For this review, take the finished solid that the model builds, in its own axes (mm). Face numbers are marked on the shaded views. A direction names the side the tool comes from. Coordinates: 2 decimals unless noted, no trailing zeros. Loops run counter-clockwise (first coordinate to the right, second up) from the corner with the lowest first, then second, coordinate; pieces in that order, holes last.
1. Machinability: for the marked faces 5 and 6, which of the approach directions +Z, -Z, +X, -X, +Y, -Y give a long, thin tool a straight path to every point of the face, cutting with its end or side? Answer none if there is none.
2. To check wall thickness, follow probe 1 along Z at (x, y) = (19, -29); probe 2 along X at (y, z) = (-30, -11); probe 3 along Z at (x, y) = (-30.5, -5.5). State the ranges of each line that lie inside material, in increasing order.
3. Clearance check with flat-ended pins moving along their axes: P1, Ø10, axis at x = -7, y = -14, coming from the -Z side; P2, Ø5, axis at x = -10.5, z = 15.5, coming from the -Y side; P3, Ø12, axis at x = -18, z = -14.5, coming from the +Y side. State where each tip first meets the part, or that it passes through.
4. Take a section at B-B, the plane z = -1.5. State the section outline as (x, y) points, then the cut area to 3 significant figures.
5. Take a section at C-C, the plane y = -28. Count the separate pieces of the cut face and the enclosed holes in it, then the cut area to 3 significant figures.
6. Mouldability with a two-part tool opening along X and no side actions: class the marked faces 1, 2, 3 and 4 as pulls with the +X half, pulls with the -X half, needs draft (parallel to the pull), parting line crosses it, or undercut.
7. Take a section at A-A, the plane x = -20. State the section outline as (y, z) points, then the cut area to 3 significant figures.
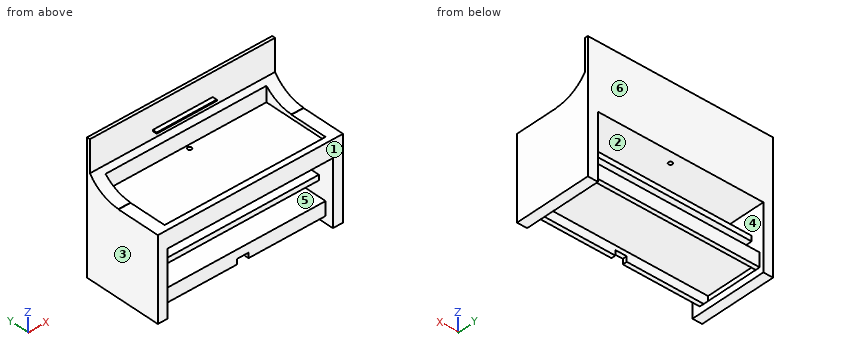
```python
from build123d import *

# Parameters (mm, degrees)
F0_W          = 109.3183457851
F0_H          = 33.4434658289
F1_DEPTH      = 45.72
F2_W          = 95.0407683849
F2_H          = 38.138333708
F3_DEPTH      = 25.4
F4_W          = 109.3183457851
F4_H          = 23.2531316578
F5_DEPTH      = 25.4
F7_DEPTH      = 254
F9_W          = 5.9644132853
F9_H          = 45.72
F9_W_2        = 5.7119317353
F10_DEPTH     = 38.1
F11_W         = 29.130092822
F11_H         = 3.0559636652
F12_DEPTH     = 101.6
F14_DEPTH     = 127
F15_DEPTH     = 18.5456499457
F16_W         = 35.4631710798
F16_H         = 0.6852131337
F17_DEPTH     = 2.54
F18_W         = 38.6509299278
F18_H         = 8.1171598285
F19_DEPTH     = 99.9768525362
F20_T         = 2.54
F20_T3_DEPTH  = 114.3983457851
F20_T5_DEPTH  = 40.5431710798
F20_T7_DEPTH  = 5.7652131337
F20_T9_DEPTH  = 12.2003224361
F20_T11_DEPTH = 12.2372549641
F20_T13_DEPTH = 50.8
F20_T15_DEPTH = 13.1971598285
F20_T17_DEPTH = 43.7309299278
F20_T19_DEPTH = 34.210092822
F20_T21_DEPTH = 8.1359636652
F20_T23_DEPTH = 7.2268683422
F20_T25_DEPTH = 43.218333708
F20_T27_DEPTH = 14.0249238314
F20_T29_DEPTH = 100.1207683849
F21_W         = 6.7161731422
F21_H         = 3.0271708965
F22_DEPTH     = 25.4
F8_R          = 1.1732121366
F23_DEPTH     = 69.3976804614


# Not quite as in the source:
# - a shell that OpenCascade refuses in one call is made with other operations: the cavity is built on its own and cut out


with BuildPart() as f1:
    # F0 (on Front) → F1 (new body)
    with BuildSketch(Plane.XZ):
        with Locations((-0.1045018435, 16.7217329144)):
            Rectangle(F0_W, F0_H)
    extrude(amount=F1_DEPTH)

    # F2 (on face) → F3 (cut)
    with BuildSketch(Plane.XY.offset(33.4434658289)):
        with Locations((-0.1229681075, -23.2116412371)):
            Rectangle(F2_W, F2_H)
    extrude(amount=-F3_DEPTH, mode=Mode.SUBTRACT)

    # F4 (on face) → F5 (cut)
    with BuildSketch(Plane.XZ.offset(45.72)):
        with Locations((-0.1045018435, 21.8169)):
            Rectangle(F4_W, F4_H)
    extrude(amount=-F5_DEPTH, mode=Mode.SUBTRACT)

    # F6 (on face) → F7 (cut)
    with BuildSketch(Plane.YZ.offset(54.5546710491)):
        with BuildLine():
            Line((-20.32, 33.4434658289), (-20.32, 10.3678972162))
            ThreePointArc((-20.32, 10.3678972162), (-8.4847772871, 13.6341404962), (0, 22.5082261516))
            Line((0, 22.5082261516), (0, 33.4434658289))
            Line((0, 33.4434658289), (-20.32, 33.4434658289))
        make_face()
        with BuildLine():
            ThreePointArc((0, 22.5082261516), (2.0560745106, 27.8049237926), (2.7555686127, 33.4434658289))
            ThreePointArc((2.7555686127, 33.4434658289), (-36.6368910458, 49.7603568747), (-20.32, 10.3678972162))
            Line((-20.32, 10.3678972162), (-20.32, 33.4434658289))
            Line((-20.32, 33.4434658289), (0, 33.4434658289))
            Line((0, 33.4434658289), (0, 22.5082261516))
        make_face()
    extrude(amount=-F7_DEPTH, mode=Mode.SUBTRACT)

    # F9 (on face) → F10 (join)
    with BuildSketch(Plane(origin=(0, 0, 0), x_dir=(1, 0, 0), z_dir=(0, 0, -1))):
        with Locations((51.5724644065, 22.86)):
            Rectangle(F9_W, F9_H)
        with Locations((-51.9077088684, 22.86)):
            Rectangle(F9_W_2, F9_H)
    extrude(amount=F10_DEPTH)

    # F11 (on face) → F12 (join)
    with BuildSketch(Plane.YZ.offset(-49.0517430007)):
        with Locations((-22.1103844233, -15.5687723309)):
            Rectangle(F11_W, F11_H)
    extrude(amount=F12_DEPTH)

    # F13 (on face) → F14 (cut)
    with BuildSketch(Plane.YZ.offset(54.5546710491)):
        with BuildLine():
            ThreePointArc((0, 22.5082261516), (-0.8668457158, 21.0315096899), (-1.8408102843, 19.6231397021))
            Line((-1.8408102843, 19.6231397021), (0, 19.6231397021))
            Line((0, 19.6231397021), (0, 22.5082261516))
        make_face()
    extrude(amount=-F14_DEPTH, mode=Mode.SUBTRACT)

    # F15 (add): a face of the model
    f15_faces = [f1.faces().sort_by_distance(p)[0] for p in [
        (-0.1045018435, -0.9204051421, 19.6231397021),
    ]]
    extrude(f15_faces, amount=F15_DEPTH)

    # F16 (on face) → F17 (join)
    with BuildSketch(Plane.XZ.offset(1.8408102843)):
        with Locations((0.1093326136, 24.1770995781)):
            Rectangle(F16_W, F16_H)
    extrude(amount=F17_DEPTH)

    # F18 (on face) → F19 (join)
    with BuildSketch(Plane(origin=(48.5902577639, 0, 0), x_dir=(0, -1, 0), z_dir=(-1, 0, 0))):
        with Locations((21.6686017811, -30.0215007737)):
            Rectangle(F18_W, F18_H)
    extrude(amount=F19_DEPTH)

    # F20: shell of thickness 2.54, made by hand


with BuildPart() as f20_core1:
    # F20_t2: copy of F1
    add(f1.part)

    # the walls: a layer under each face that stays
    f20_faces = [f20_core1.faces().sort_by_distance(p)[0] for p in [
        (-54.763674736, -22.86, 0.0343948239),
        (-0.1045018435, 0, 0.0343948239),
        (-0.1045018435, -0.9204051421, 38.1687896479),
        (-0.1045018435, -1.8408102843, 28.895964675),
        (-46.9552214657, -2.7975084588, 18.4286678952),
        (-51.203513518, -20.32, 10.2791156936),
        (-46.9552214657, -43.9057142857, 10.1903341711),
        (-36.5439504385, -45.72, 2.1419451425),
        (-51.9077088684, -22.86, -38.1),
        (54.5546710491, -22.86, 0.0343948239),
        (-49.0517430007, -22.86, -19.05),
        (-0.2307426184, -22.86, 0),
        (48.5902577639, -22.86, -19.05),
        (51.5724644065, -22.86, -38.1),
        (0.1093326136, -3.1108102843, 24.5197061449),
        (-17.6222529262, -3.1108102843, 24.1770995781),
        (0.1093326136, -3.1108102843, 23.8344930112),
        (17.8409181535, -3.1108102843, 24.1770995781),
        (-47.6433522999, -10.4988633345, 9.5342864675),
        (-0.1229681075, -4.1424743831, 12.5159277446),
        (47.397416085, -35.9244191398, 9.5342864675),
        (50.9760435671, -20.32, 10.2791156936),
        (-0.1229681075, -42.2808080912, 9.1169),
        (-0.2307426184, -40.994066745, -30.0215007737),
        (-0.2307426184, -21.6686017811, -25.9629208595),
        (-0.2307426184, -2.3431368172, -30.0215007737),
        (-0.2307426184, -22.1103844233, -14.0407904983),
        (-0.2307426184, -7.5453380123, -15.5687723309),
        (-0.2307426184, -36.6754308343, -15.5687723309),
        (-0.2307426184, -22.1103844233, -17.0967541635),
        (0.1093326136, -4.3808102843, 24.1770995781),
        (-0.1229681075, -23.2116412371, 8.0434658289),
    ]]
    thicken(f20_faces, amount=-F20_T, mode=Mode.SUBTRACT)

    # F20_s4 → F20_t3 (cut)
    with BuildSketch(Plane.YZ.offset(-57.303674736)):
        Polygon((-1.8865509063, 19.6383521673), (0.6991897157, 19.6231397021), (0.6991897157, 18.7783837759), (0.1932519166, 18.1018931859), align=None)
    extrude(amount=F20_T3_DEPTH, mode=Mode.SUBTRACT)

    # F20_s6 → F20_t5 (cut)
    with BuildSketch(Plane.YZ.offset(-20.1622529262)):
        Polygon((-1.8662102843, 24.5451061449), (0.6991897157, 24.5197061449), (0.6991897157, 21.9797061449), (-1.8408102843, 21.9797061449), align=None)
        Polygon((-1.8662102843, 23.8090930112), (0.6991897157, 23.8344930112), (0.6991897157, 26.3744930112), (-1.8408102843, 26.3744930112), align=None)
    extrude(amount=F20_T5_DEPTH, mode=Mode.SUBTRACT)

    # F20_s8 → F20_t7 (cut)
    with BuildSketch(Plane.XY.offset(21.2944930112)):
        Polygon((-17.6476529262, -1.8662102843), (-17.6222529262, 0.6991897157), (-15.0822529262, 0.6991897157), (-15.0822529262, -1.8408102843), align=None)
        Polygon((17.8663181535, -1.8662102843), (17.8409181535, 0.6991897157), (15.3009181535, 0.6991897157), (15.3009181535, -1.8408102843), align=None)
    extrude(amount=F20_T7_DEPTH, mode=Mode.SUBTRACT)

    # F20_s10 → F20_t9 (cut)
    with BuildSketch(Plane.YZ.offset(-57.303674736)):
        Polygon((-20.3454, 10.2157341711), (-17.78, 10.1903341711), (-17.78, 7.6503341711), (-20.32, 7.6503341711), align=None)
    extrude(amount=F20_T9_DEPTH, mode=Mode.SUBTRACT)

    # F20_s12 → F20_t11 (cut)
    with BuildSketch(Plane.YZ.offset(44.857416085)):
        Polygon((-20.3454, 10.2157341711), (-20.32, 7.6503341711), (-17.78, 7.6503341711), (-17.78, 10.1903341711), align=None)
    extrude(amount=F20_T11_DEPTH, mode=Mode.SUBTRACT)

    # F20_s14 → F20_t13 (cut)
    with BuildSketch(Plane.XZ.offset(-2.54)):
        Polygon((-49.0263430007, -0.0254), (-51.5917430007, 0), (-51.5917430007, 2.54), (-49.0517430007, 2.54), align=None)
        Polygon((48.5648577639, -0.0254), (48.5902577639, 2.54), (51.1302577639, 2.54), (51.1302577639, 0), align=None)
    extrude(amount=F20_T13_DEPTH, mode=Mode.SUBTRACT)

    # F20_s16 → F20_t15 (cut)
    with BuildSketch(Plane.XY.offset(-36.620080688)):
        Polygon((-49.0263430007, -41.019466745), (-51.5917430007, -40.994066745), (-51.5917430007, -38.454066745), (-49.0517430007, -38.454066745), align=None)
        Polygon((-49.0263430007, -2.3177368172), (-51.5917430007, -2.3431368172), (-51.5917430007, -4.8831368172), (-49.0517430007, -4.8831368172), align=None)
        Polygon((48.5648577639, -2.3177368172), (51.1302577639, -2.3431368172), (51.1302577639, -4.8831368172), (48.5902577639, -4.8831368172), align=None)
        Polygon((48.5648577639, -41.019466745), (51.1302577639, -40.994066745), (51.1302577639, -38.454066745), (48.5902577639, -38.454066745), align=None)
    extrude(amount=F20_T15_DEPTH, mode=Mode.SUBTRACT)

    # F20_s18 → F20_t17 (cut)
    with BuildSketch(Plane.XZ.offset(-0.1968631828)):
        Polygon((-49.0263430007, -25.9375208595), (-51.5917430007, -25.9629208595), (-51.5917430007, -28.5029208595), (-49.0517430007, -28.5029208595), align=None)
        Polygon((48.5648577639, -25.9375208595), (51.1302577639, -25.9629208595), (51.1302577639, -28.5029208595), (48.5902577639, -28.5029208595), align=None)
    extrude(amount=F20_T17_DEPTH, mode=Mode.SUBTRACT)

    # F20_s20 → F20_t19 (cut)
    with BuildSketch(Plane.XZ.offset(5.0053380123)):
        Polygon((-49.0263430007, -14.0153904983), (-51.5917430007, -14.0407904983), (-51.5917430007, -16.5807904983), (-49.0517430007, -16.5807904983), align=None)
        Polygon((-49.0263430007, -17.1221541635), (-51.5917430007, -17.0967541635), (-51.5917430007, -14.5567541635), (-49.0517430007, -14.5567541635), align=None)
        Polygon((48.5648577639, -17.1221541635), (51.1302577639, -17.0967541635), (51.1302577639, -14.5567541635), (48.5902577639, -14.5567541635), align=None)
        Polygon((48.5648577639, -14.0153904983), (51.1302577639, -14.0407904983), (51.1302577639, -16.5807904983), (48.5902577639, -16.5807904983), align=None)
    extrude(amount=F20_T19_DEPTH, mode=Mode.SUBTRACT)

    # F20_s22 → F20_t21 (cut)
    with BuildSketch(Plane.XY.offset(-19.6367541635)):
        Polygon((-49.0263430007, -7.5199380123), (-51.5917430007, -7.5453380123), (-51.5917430007, -10.0853380123), (-49.0517430007, -10.0853380123), align=None)
        Polygon((-49.0263430007, -36.7008308343), (-51.5917430007, -36.6754308343), (-51.5917430007, -34.1354308343), (-49.0517430007, -34.1354308343), align=None)
        Polygon((48.5648577639, -7.5199380123), (51.1302577639, -7.5453380123), (51.1302577639, -10.0853380123), (48.5902577639, -10.0853380123), align=None)
        Polygon((48.5648577639, -36.7008308343), (51.1302577639, -36.6754308343), (51.1302577639, -34.1354308343), (48.5902577639, -34.1354308343), align=None)
    extrude(amount=F20_T21_DEPTH, mode=Mode.SUBTRACT)

    # F20_s24 → F20_t23 (cut)
    with BuildSketch(Plane.XY.offset(5.5034658289)):
        Polygon((-47.6179522999, -42.2554080912), (-50.1833522999, -42.2808080912), (-50.1833522999, -44.8208080912), (-47.6433522999, -44.8208080912), align=None)
        Polygon((47.372016085, -42.2554080912), (49.937416085, -42.2808080912), (49.937416085, -44.8208080912), (47.397416085, -44.8208080912), align=None)
    extrude(amount=F20_T23_DEPTH, mode=Mode.SUBTRACT)

    # F20_s26 → F20_t25 (cut)
    with BuildSketch(Plane.XZ.offset(1.6024743831)):
        Polygon((-47.6179522999, 8.0688658289), (-50.1833522999, 8.0434658289), (-50.1833522999, 5.5034658289), (-47.6433522999, 5.5034658289), align=None)
        Polygon((47.372016085, 8.0688658289), (49.937416085, 8.0434658289), (49.937416085, 5.5034658289), (47.397416085, 5.5034658289), align=None)
    extrude(amount=F20_T25_DEPTH, mode=Mode.SUBTRACT)

    # F20_s28 → F20_t27 (cut)
    with BuildSketch(Plane.XY.offset(5.5034658289)):
        Polygon((-47.6179522999, -4.1678743831), (-50.1833522999, -4.1424743831), (-50.1833522999, -1.6024743831), (-47.6433522999, -1.6024743831), align=None)
        Polygon((47.372016085, -4.1678743831), (47.397416085, -1.6024743831), (49.937416085, -1.6024743831), (49.937416085, -4.1424743831), align=None)
    extrude(amount=F20_T27_DEPTH, mode=Mode.SUBTRACT)

    # F20_s30 → F20_t29 (cut)
    with BuildSketch(Plane.YZ.offset(-50.1833522999)):
        Polygon((-4.1678743831, 8.0688658289), (-1.6024743831, 8.0434658289), (-1.6024743831, 5.5034658289), (-4.1424743831, 5.5034658289), align=None)
        Polygon((-42.2554080912, 8.0688658289), (-44.8208080912, 8.0434658289), (-44.8208080912, 5.5034658289), (-42.2808080912, 5.5034658289), align=None)
    extrude(amount=F20_T29_DEPTH, mode=Mode.SUBTRACT)


with BuildPart() as f1_1:
    add(f1.part)

    # what is left inside the walls is the cavity
    f20_cavity = [f20_core1.part.solids().sort_by_distance(p)[0] for p in [
        (-0.230743, -29.633333, 2.5654),
    ]]
    add(f20_cavity, mode=Mode.SUBTRACT)

    # F21 (on face) → F22 (cut)
    with BuildSketch(Plane.XZ.offset(40.994066745)):
        with Locations((-0.2307426184, -32.5664952397)):
            Rectangle(F21_W, F21_H)
    extrude(amount=-F22_DEPTH, mode=Mode.SUBTRACT)

    # F8 (on face) → F23 (cut)
    with BuildSketch(Plane.XY.offset(8.0434658289)):
        with Locations((0, -6.3559673727)):
            Circle(F8_R)
    extrude(amount=-F23_DEPTH, mode=Mode.SUBTRACT)


solid = f1_1.part
```
Results list:
1. face 5: +Y, -Y
1. face 6: +Z, -Z, +X, -X, +Y
2. probe 1: z = -28.5 to -25.96, -17.1 to -14.04, 0 to 2.54, 5.5 to 8.04
2. probe 2: x = -54.76 to -52.22, -51.59 to -49.05, 48.59 to 51.13, 52.01 to 54.55
2. probe 3: z = -28.5 to -25.96, 0 to 2.54, 5.5 to 8.04
3. P1: stops at z = -28.5
3. P2: stops at y = -4.14
3. P3: stops at y = -7.55
4. outline: (-54.76, -45.72) - (-49.05, -45.72) - (-49.05, 0) - (-54.76, 0) - close; (48.59, -45.72) - (54.55, -45.72) - (54.55, 0) - (48.59, 0) - close; hole (-52.22, -43.18) - (-51.59, -43.18) - (-51.59, -2.54) - (-52.22, -2.54) - close; hole (51.13, -43.18) - (52.01, -43.18) - (52.01, -2.54) - (51.13, -2.54) - close
4. area: 472 mm2
5. separate pieces: 2
5. enclosed holes: 2
5. area: 1,500 mm2
6. face 1: needs draft
6. face 2: undercut
6. face 3: pulls with the -X half
6. face 4: undercut
7. outline: (-45.72, 0) - (0, 0) - (0, 38.17) - (-1.84, 38.17) - (-1.84, 19.62) arc R23.08 cw to (-4.14, 16.99) - (-4.14, 8.04) - (-42.28, 8.04) - (-42.28, 10.19) - (-45.72, 10.19) - close; (-40.99, -34.08) - (-38.45, -34.08) - (-38.45, -28.5) - (-4.88, -28.5) - (-4.88, -34.08) - (-2.34, -34.08) - (-2.34, -25.96) - (-40.99, -25.96) - close; (-36.68, -17.1) - (-7.55, -17.1) - (-7.55, -14.04) - (-36.68, -14.04) - close; hole (-43.18, 2.54) - (-2.54, 2.54) - (-2.54, 5.5) - (-43.18, 5.5) - close
7. area: 549 mm2
